Part model, mm, in its own coordinate system. A direction names the side the tool comes from. Coordinates: 2 decimals unless noted, no trailing zeros. Loops run counter-clockwise (first coordinate to the right, second up) from the corner with the lowest first, then second, coordinate; pieces in that order, holes last. Notation, with made-up numbers: M 79.5,24 L 83.5,24 A18 ccw 83.5,53 Z; hole C 29.25,69 d3. An arc over 180 degrees is marked long. Use a Markdown table: item, result. Add a question column.
1) Band-saw the part on A-A (x = 313). List the corners of the cut face in (y, z).
2) Tool access for faces 1 (the flat face through (155, -9, 230)), 2 (the cylindrical face through (425.72, -18.1, 78.99)), 3 (the cylindrical face through (425.72, -0.9, 78.99)): list every direction of +Z, -Z, +X, -X, +Y, -Y with a clear straight run to the whole face (end or side of a thin tool).
3) Pull direction X, two halves, no side cores. Call faces 4 (the flat face through (478.589, -9.409, 85.877)), 5 (the cylindrical face through (127.49, -9.41, 181.47)), 6 (the cylindrical face through (29.1, -0.9, 113.18)), 7 (the flat face through (231, -19, 198)): released by +X, released by -X, zero draft, split by the parting line, or undercut.
4) Pin check, flat tips, straight feed: pin 1 Ø11 at (y, z) = (-8, 233) entering from -X; pin 2 Ø2 at (y, z) = (-12.5, 31) entering from -X; pin 3 Ø2 at (x, y) = (160.5, -14.5) entering from -Z. Stop position of each tip, or through.
5) Wall check: probe 1 along Z at (x, y) = (228.5, -4.5); probe 2 along Z at (x, y) = (300, -4.5); probe 3 along X at (y, z) = (-4, 143). Give the ranges that are in metal, low to high. Write a range as from..to.
6) Band-saw the part on B-B (y = -7.5). List the corners of the cut face in (x, z).
from build123d import *

# Parameters (mm, degrees)
F1_DEPTH = 19
F2_R     = 3


with BuildPart() as f1:
    # F0 (on Front) → F1 (new body)
    with BuildSketch(Plane.XZ):
        with BuildLine():
            Line((57.345441, 230), (0, 0))
            Line((0, 0), (41.681786, 0))
            Line((41.681786, 0), (109.401036, 159.536556))
            ThreePointArc((109.401036, 159.536556), (127.82943, 181.694291), (155.426279, 190))
            Line((155.426279, 190), (250, 190))
            Line((250, 190), (344.573721, 190))
            ThreePointArc((344.573721, 190), (372.17057, 181.694291), (390.598964, 159.536556))
            Line((390.598964, 159.536556), (458.318214, 0))
            Line((458.318214, 0), (500, 0))
            Line((500, 0), (456.569009, 174.19219))
            ThreePointArc((456.569009, 174.19219), (421.105584, 228.801075), (359.539437, 250))
            Line((359.539437, 250), (260, 250))
            ThreePointArc((260, 250), (252.928932, 247.071068), (250, 240))
            Line((250, 240), (250, 230))
            Line((250, 230), (57.345441, 230))
        make_face()
    extrude(amount=F1_DEPTH)

    # F2
    f2_edges = [f1.edges().sort_by_distance(p)[0] for p in [
        (28.67272, -19, 115),
        (20.840893, -19, 0),
        (75.541411, -19, 79.768278),
        (127.82943, -19, 181.694291),
        (250, -19, 190),
        (372.17057, -19, 181.694291),
        (424.458589, -19, 79.768278),
        (479.159107, -19, 0),
        (478.284505, -19, 87.096095),
        (421.105584, -19, 228.801075),
        (309.769718, -19, 250),
        (252.928932, -19, 247.071068),
        (250, -19, 235),
        (153.67272, -19, 230),
        (28.67272, 0, 115),
        (20.840893, 0, 0),
        (75.541411, 0, 79.768278),
        (127.82943, 0, 181.694291),
        (250, 0, 190),
        (372.17057, 0, 181.694291),
        (424.458589, 0, 79.768278),
        (479.159107, 0, 0),
        (478.284505, 0, 87.096095),
        (421.105584, 0, 228.801075),
        (309.769718, 0, 250),
        (252.928932, 0, 247.071068),
        (250, 0, 235),
        (153.67272, 0, 230),
    ]]
    fillet(f2_edges, radius=F2_R)


solid = f1.part
Entries:
| question | item | result |
|---|---|---|
| 1 | outline | M -19,193 A3 ccw -16,190 L -3,190 A3 ccw 0,193 L 0,247 A3 ccw -3,250 L -16,250 A3 ccw -19,247 Z |
| 2 | face 1 | +Z, -X, +Y, -Y |
| 2 | face 2 | -Z, -Y |
| 2 | face 3 | -Z, +Y |
| 3 | face 4 | released by +X |
| 3 | face 5 | undercut |
| 3 | face 6 | released by -X |
| 3 | face 7 | zero draft |
| 4 | pin 1 | x = 56.72 |
| 4 | pin 2 | x = 7.48 |
| 4 | pin 3 | z = 190 |
| 5 | probe 1 | 190..230 |
| 5 | probe 2 | 190..250 |
| 5 | probe 3 | 35.65..102.38, 397.62..464.35 |
| 6 | outline | M 0,0 L 41.68,0 L 109.4,159.54 A50 cw 155.43,190 L 344.57,190 A50 cw 390.6,159.54 L 458.32,0 L 500,0 L 456.57,174.19 A100 ccw 359.54,250 L 260,250 A10 ccw 250,240 L 250,230 L 57.35,230 Z |
